```python
from build123d import *

# Parameters (mm, degrees)
SKETCH1_W           = 115
SKETCH1_H           = 60
SKETCH1_R           = 2.1
BOSS_EXTRUDE2_DEPTH = 7
SKETCH2_R           = 4
CUT_EXTRUDE1_DEPTH  = 3
SKETCH5_W           = 8.5
SKETCH5_H           = 8.5
BOSS_EXTRUDE3_DEPTH = 25
SKETCH6_R           = 1.75
CUT_EXTRUDE2_DEPTH  = 10


with BuildPart() as part:
    # Sketch1 → Boss-Extrude2 (new body)
    with BuildSketch(Plane(origin=(0, 0, 0), x_dir=(1, 0, 0), z_dir=(0, 1, 0))):
        with Locations((57.5, 30)):
            Rectangle(SKETCH1_W, SKETCH1_H)
        with Locations(Location((57.5, 30, 0), (0, 0, 270))):
            Circle(SKETCH1_R, mode=Mode.SUBTRACT)
        with Locations(Location((12.5, 30, 0), (0, 0, 270))):
            Circle(SKETCH1_R, mode=Mode.SUBTRACT)
        with Locations(Location((102.5, 30, 0), (0, 0, 90))):
            Circle(SKETCH1_R, mode=Mode.SUBTRACT)
    extrude(amount=BOSS_EXTRUDE2_DEPTH)

    # Sketch2 → Cut-Extrude1 (cut)
    with BuildSketch(Plane(origin=(0, 7, 0), x_dir=(1, 0, 0), z_dir=(0, 1, 0))):
        with Locations(Location((12.5, 30, 0), (0, 0, 270))):
            Circle(SKETCH2_R)
        with Locations(Location((57.5, 30, 0), (0, 0, 270))):
            Circle(SKETCH2_R)
        with Locations(Location((102.5, 30, 0), (0, 0, 270))):
            Circle(SKETCH2_R)
    extrude(amount=-CUT_EXTRUDE1_DEPTH, mode=Mode.SUBTRACT)

    # Sketch5 → Boss-Extrude3 (add)
    with BuildSketch(Plane(origin=(0, 7, 0), x_dir=(1, 0, 0), z_dir=(0, 1, 0))):
        with Locations((19.25, 53.75)):
            Rectangle(SKETCH5_W, SKETCH5_H)
        with Locations((19.25, 6.25)):
            Rectangle(SKETCH5_W, SKETCH5_H)
        Polygon((73, 58), (77.25, 58), (81.5, 58), (81.5, 49.5), (73, 49.5), align=None)
        Polygon((73, 10.5), (73, 2), (77.25, 2), (81.5, 2), (81.5, 10.5), align=None)
    extrude(amount=BOSS_EXTRUDE3_DEPTH)

    # Sketch6 → Cut-Extrude2 (cut)
    with BuildSketch(Plane(origin=(0, 32, 0), x_dir=(1, 0, 0), z_dir=(0, 1, 0))):
        with Locations(Location((19.25, 53.75, 0), (0, 0, 270))):
            Circle(SKETCH6_R)
        with Locations(Location((77.25, 53.75, 0), (0, 0, 270))):
            Circle(SKETCH6_R)
        with Locations(Location((19.25, 6.25, 0), (0, 0, 270))):
            Circle(SKETCH6_R)
        with Locations(Location((77.25, 6.25, 0), (0, 0, 270))):
            Circle(SKETCH6_R)
    extrude(amount=-CUT_EXTRUDE2_DEPTH, mode=Mode.SUBTRACT)


solid = part.part
```
Part model, mm, in its own coordinate system. A direction names the side the tool comes from. Round coordinates to 2 decimals unless told otherwise and drop trailing zeros. Loops run counter-clockwise (first coordinate to the right, second up) from the corner with the lowest first, then second, coordinate; pieces in that order, holes last. Notation, with made-up numbers: (78.5, 18.25) -> (115.5, 18.25) arc R28 cw to (115.5, 45.25) -> close; hole circle Ø9 at (16.5, -7). An arc over 180 degrees is marked (long way). Use one line per item in the form item = value. Start each with the question number.
Item 1: Drill centre lines: line 1 along X through (y, z) = (6, -30); line 2 along X through (y, z) = (2.1, -30); line 3 along Z through (x, y) = (77.25, 27.75). Where is each one in solid material? Low to high.
Item 2: Two-plate mould, pull along X, no slides. Class faces 5 (the flat face through (23.5, 19, -6)), 6 (the flat face through (0, 3, -30)), 7 (the flat face through (75, 32, -54)): released by +X, released by -X, zero draft, split by the parting line, or undercut.
Item 3: Band-saw the part on C-C (x = 102.5). List the corners of the cut face in (y, z).
Item 4: Band-saw the part on B-B (z = -30). List the corners of the cut face in (x, y), plus the area to 3 significant figures.
Item 5: Drop flat-ended pins along their axis: pin 1 Ø1 at (x, z) = (76.5, -5.5) entering from +Y; pin 2 Ø2.5 at (y, z) = (14, -5) entering from -X; pin 3 Ø4 at (x, z) = (56, -30) entering from +Y. Give the stop position or say it passes through.
Item 6: Band-saw the part on A-A (y = 12). List the corners of the cut face in (x, z), plus the area to 3 significant figures.
Item 7: Tool access for faces 1 (the flat face through (77, 19, -10.5)), 2 (the flat face through (73, 19, -54)), 3 (the flat face through (77, 22, -6)), 4 (the flat face through (15, 19, -6)): list every direction of +Z, -Z, +X, -X, +Y, -Y with a clear straight run to the whole face (end or side of a thin tool).
Item 8: Band-saw the part on D-D (z = -6.25). List the corners of the cut face in (x, y).
Data:
q1.line_1 = 0 to 8.5, 16.5 to 53.5, 61.5 to 98.5, 106.5 to 115
q1.line_2 = 0 to 10.4, 14.6 to 55.4, 59.6 to 100.4, 104.6 to 115
q1.line_3 = -58 to -55.5, -52 to -49.5, -10.5 to -8, -4.5 to -2
q2.face_5 = undercut
q2.face_6 = released by -X
q2.face_7 = zero draft
q3.outline = (0, -60) -> (7, -60) -> (7, -34) -> (4, -34) -> (4, -32.1) -> (0, -32.1) -> close; (0, -27.9) -> (4, -27.9) -> (4, -26) -> (7, -26) -> (7, 0) -> (0, 0) -> close
q4.outline = (0, 0) -> (10.4, 0) -> (10.4, 4) -> (8.5, 4) -> (8.5, 7) -> (0, 7) -> close; (14.6, 0) -> (55.4, 0) -> (55.4, 4) -> (53.5, 4) -> (53.5, 7) -> (16.5, 7) -> (16.5, 4) -> (14.6, 4) -> close; (59.6, 0) -> (100.4, 0) -> (100.4, 4) -> (98.5, 4) -> (98.5, 7) -> (61.5, 7) -> (61.5, 4) -> (59.6, 4) -> close; (104.6, 0) -> (115, 0) -> (115, 7) -> (106.5, 7) -> (106.5, 4) -> (104.6, 4) -> close
q4.area = 683 mm^2
q5.pin_1 = 22
q5.pin_2 = 15
q5.pin_3 = 4
q6.outline = (15, -58) -> (23.5, -58) -> (23.5, -49.5) -> (15, -49.5) -> close; (15, -10.5) -> (23.5, -10.5) -> (23.5, -2) -> (15, -2) -> close; (73, -58) -> (81.5, -58) -> (81.5, -49.5) -> (73, -49.5) -> close; (73, -10.5) -> (81.5, -10.5) -> (81.5, -2) -> (73, -2) -> close
q6.area = 289 mm^2
q7.face_1 = +X, -X, +Y
q7.face_2 = +Z, -Z, +Y
q7.face_3 = +Y
q7.face_4 = +Z, -Z, -X, +Y
q8.outline = (0, 0) -> (115, 0) -> (115, 7) -> (81.5, 7) -> (81.5, 32) -> (79, 32) -> (79, 22) -> (75.5, 22) -> (75.5, 32) -> (73, 32) -> (73, 7) -> (23.5, 7) -> (23.5, 32) -> (21, 32) -> (21, 22) -> (17.5, 22) -> (17.5, 32) -> (15, 32) -> (15, 7) -> (0, 7) -> close
